```python
from build123d import *

# Parameters (mm, degrees)
F0_R     = 7.875
F1_DEPTH = 0.25
F2_W     = 1
F2_H     = 2
F3_DEPTH = 0.5
F5_DEPTH = 0.5
F7_DEPTH = 1


# Not quite as in the source:
# - a feature names something its author has since deleted; it is built from what else it names


with BuildPart() as f1:
    # F0 (on Top) → F1 (new body)
    with BuildSketch(Plane.XY):
        Circle(F0_R)
    extrude(amount=F1_DEPTH)

    # F2 (on face) → F3 (join)
    with BuildSketch(Plane.XY.offset(0.25)):
        with Locations((-1, 0)):
            Rectangle(F2_W, F2_H)
        with Locations((1, 0)):
            Rectangle(F2_W, F2_H)
    extrude(amount=F3_DEPTH)

    # F4 (on face) → F5 (cut)
    with BuildSketch(Plane.XY.offset(0.25)):
        with BuildLine():
            ThreePointArc((-0.5, -7.8591109548), (0, -7.875), (0.5, -7.8591109548))
            Line((0.5, -7.8591109548), (0.5, -7.125))
            ThreePointArc((0.5, -7.125), (0.4267766953, -6.9482233047), (0.25, -6.875))
            Line((0.25, -6.875), (-0.25, -6.875))
            ThreePointArc((-0.25, -6.875), (-0.4267766953, -6.9482233047), (-0.5, -7.125))
            Line((-0.5, -7.125), (-0.5, -7.8591109548))
        make_face()
    extrude(amount=-F5_DEPTH, mode=Mode.SUBTRACT)

    # F6 (on face) → F7 (cut)
    with BuildSketch(Plane.XY.offset(0.25)):
        with BuildLine():
            ThreePointArc((-5.2149125113, 5.2149125113), (-6.8136115523, 2.8222903137), (-7.375, 0))
            ThreePointArc((-7.375, 0), (-7.625, -0.25), (-7.875, 0))
            ThreePointArc((-7.875, 0), (-7.8628378306, -0.4375), (-7.8263888889, -0.8736486478))
            ThreePointArc((-7.8263888889, -0.8736486478), (-7.2393272374, -0.6012862371), (-7, 0))
            ThreePointArc((-7, 0), (-6.4671567276, 2.6787840266), (-4.9497474683, 4.9497474683))
            ThreePointArc((-4.9497474683, 4.9497474683), (-4.9497474683, 5.2149125113), (-5.2149125113, 5.2149125113))
        make_face()
        with BuildLine():
            ThreePointArc((7.875, 0), (7.8628378306, 0.4375), (7.8263888889, 0.8736486478))
            ThreePointArc((7.8263888889, 0.8736486478), (7.2393272374, 0.6012862371), (7, 0))
            ThreePointArc((7, 0), (6.4671567276, -2.6787840266), (4.9497474683, -4.9497474683))
            ThreePointArc((4.9497474683, -4.9497474683), (4.9497474683, -5.2149125113), (5.2149125113, -5.2149125113))
            ThreePointArc((5.2149125113, -5.2149125113), (6.8136115523, -2.8222903137), (7.375, 0))
            ThreePointArc((7.375, 0), (7.625, 0.25), (7.875, 0))
        make_face()
    extrude(amount=-F7_DEPTH, mode=Mode.SUBTRACT)


solid = f1.part
```
Geometry check sheet. Reference: the model listing, model coordinates, mm. Give positions to 0.01 mm unless a question says otherwise; leave off trailing zeros. Order: outer loops, then holes, each group sorted by start corner. A loop starts at its lowest first (then second) coordinate and runs counter-clockwise, first axis right, second up. Notation, with made-up numbers: (36.5, 83.5) - (45.5, 83.5) arc R20 ccw to (45.5, 92.5) - close; hole circle Ø1 at (-6, 71.25). An arc over 180 degrees is marked (long way). Answer in a Markdown table with one row per item. Add a question column.
Q1. Cross-section at C-C, the plane x = 0. Enter the section's corners in (y, z) (3 decimals).
Q2. Cross-section at A-A, the plane z = 0.4. Enter the section's corners in (x, y), then the cut area to 3 significant figures.
Q3. Material ranges on probe 1 along X at (y, z) = (0, 0.55); probe 2 along Z at (x, y) = (4, 5.25); probe 3 along X at (y, z) = (-2.75, 0.15), recorded low to high. Write a range as from..to.
Q4. Cross-section at B-B, the plane y = -4.75. Enter the section's corners in (x, z).
Q5. Cross-section at D-D, the plane y = 6. Enter the section's corners in (x, z), then the cut area to 3 significant figures.
Check values:
| question | item | result |
|---|---|---|
| 1 | outline | (-6.875, 0) - (7.875, 0) - (7.875, 0.25) - (-6.875, 0.25) - close |
| 2 | outline | (-1.5, -1) - (-0.5, -1) - (-0.5, 1) - (-1.5, 1) - close; (0.5, -1) - (1.5, -1) - (1.5, 1) - (0.5, 1) - close |
| 2 | area | 4.00 mm^2 |
| 3 | probe 1 | x = -1.5..-0.5, 0.5..1.5 |
| 3 | probe 2 | z = 0..0.25 |
| 3 | probe 3 | x = -7.38..6.44, 6.84..7.38 |
| 4 | outline | (-6.28, 0) - (5.14, 0) - (5.14, 0.25) - (-6.28, 0.25) - close; (5.64, 0) - (6.28, 0) - (6.28, 0.25) - (5.64, 0.25) - close |
| 5 | outline | (-5.1, 0) - (5.1, 0) - (5.1, 0.25) - (-5.1, 0.25) - close |
| 5 | area | 2.55 mm^2 |
